Build history of the part. All positions in model axes, mm. A direction names the side the tool comes from. Give positions to 0.01 mm unless a question says otherwise; leave off trailing zeros. Order: outer loops, then holes, each group sorted by start corner. A loop starts at its lowest first (then second) coordinate and runs counter-clockwise, first axis right, second up. Notation, with made-up numbers: M -19.75,43 L 3.25,43 A22 ccw 3.25,80 Z; hole C 34.5,21.5 d10. An arc over 180 degrees is marked long. One line per item, written item: value. Start each with the question number.
from build123d import *

# Parameters (mm, degrees)
BOSS_EXTRUDE1_DEPTH = 368
SHELL2_T            = -3
BOSS_EXTRUDE3_REACH = 402.691
CUT_EXTRUDE1_REACH  = 402.691
SKETCH9_R           = 20
BOSS_EXTRUDE4_START = 10
SKETCH10_R          = 21.5
SKETCH10_R_2        = 20
BOSS_EXTRUDE4_DEPTH = 10
SKETCH11_W          = 368
SKETCH11_H          = 246
SKETCH11_W_2        = 362
SKETCH11_H_2        = 240
BOSS_EXTRUDE5_DEPTH = 38


with BuildPart() as part:
    # Sketch2 → Boss-Extrude1 (new body)
    with BuildSketch(Plane(origin=(0, 0, 0), x_dir=(0, 0, -1), z_dir=(1, 0, 0))):
        Polygon((123, -50), (-123, -50), (-52.5, 100), (52.5, 100), align=None)
    extrude(amount=BOSS_EXTRUDE1_DEPTH)

    # Shell2
    shell2_openings = [part.faces().sort_by_distance(p)[0] for p in [
        (184, 100, 0),
        (184, -50, 0),
    ]]
    offset(amount=SHELL2_T, openings=shell2_openings, kind=Kind.INTERSECTION)

    # Sketch8 → Boss-Extrude3 (add, up to next)
    with BuildSketch(Plane(origin=(368, 0, 0), x_dir=(0, 0, -1), z_dir=(1, 0, 0)), mode=Mode.PRIVATE) as boss_extrude3_sk1:
        Polygon((-4.5, 100), (-30, -35), (30, -35), (4.5, 100), (1.5, 100), (26.433333333, -32), (-26.433333333, -32), (-1.5, 100), align=None)
    boss_extrude3_tool1 = extrude(boss_extrude3_sk1.sketch, amount=-BOSS_EXTRUDE3_REACH, mode=Mode.PRIVATE) - part.part
    add(boss_extrude3_tool1.solids().sort_by_distance((368, 34.274202, 15.418325))[0])

    # Sketch9 → Cut-Extrude1 (cut, up to next)
    with BuildSketch(Plane(origin=(368, 0, 0), x_dir=(0, 0, -1), z_dir=(1, 0, 0)), mode=Mode.PRIVATE) as cut_extrude1_sk1:
        with Locations((0, -10)):
            Circle(SKETCH9_R)
    cut_extrude1_tool1 = extrude(cut_extrude1_sk1.sketch, amount=-CUT_EXTRUDE1_REACH, mode=Mode.PRIVATE) & part.part
    add(cut_extrude1_tool1.solids().sort_by_distance((368, -10, 0))[0], mode=Mode.SUBTRACT)

    # Sketch10 → Boss-Extrude4 (add)
    with BuildSketch(Plane(origin=(368, 0, 0), x_dir=(0, 0, -1), z_dir=(1, 0, 0)).offset(BOSS_EXTRUDE4_START)):
        with Locations(Location((0, -10, 0), (0, 0, 180))):
            Circle(SKETCH10_R)
        with Locations((0, -10)):
            Circle(SKETCH10_R_2, mode=Mode.SUBTRACT)
    extrude(amount=-BOSS_EXTRUDE4_DEPTH)

    # Sketch11 → Boss-Extrude5 (add)
    with BuildSketch(Plane.XZ.offset(50)):
        with Locations((184, 0)):
            Rectangle(SKETCH11_W, SKETCH11_H)
        with Locations((184, 0)):
            Rectangle(SKETCH11_W_2, SKETCH11_H_2, mode=Mode.SUBTRACT)
    extrude(amount=BOSS_EXTRUDE5_DEPTH)


solid = part.part
1) Tool access for faces 5 (the flat face through (187, -35, 0)), 6 (the flat face through (3, 20, 0)), 7 (the cylindrical face through (371.591, -27.743, -9.229)), 8 (the flat face through (378, 3, 16)), 9 (the flat face through (186.534, 31.555, -17.428)): list every direction of +Z, -Z, +X, -X, +Y, -Y with a clear straight run to the whole face (end or side of a thin tool).
2) Drop flat-ended pins along their axis: P1, Ø1, axis at y = 31.5, z = 72.5, coming from the +X side; P2, Ø1, axis at x = 196.5, y = 49, coming from the +Z side (3 decimals); P3, Ø6, axis at x = 335, y = -0.5, coming from the +Z side (3 decimals). Give the stop position or say it passes through.
3) Slice it at B-B (y = 77.5). List the corners of the cut face in (x, z) (3 decimals), plus the area to 3 significant figures.
4) Slice it at A-A (x = 167.5). List the corners of the cut face in (y, z), plus the area to 3 significant figures.
5) Slice it at D-D (y = 2). List the corners of the cut face in (x, z), plus the area to 3 significant figures.
6) Slice it at C-C (z = 84). List the corners of the cut face in (x, y), plus the area to 3 significant figures.
7) Drill centre lines: line 1 (X direction, y = -21, z = -97); line 2 (Y direction, x = 373, z = 0); line 3 (Z direction, x = 45, y = -73). Where is each one in solid material? Low to high.
8) Pull direction X, two halves, no side cores. Call faces 1 (the flat face through (365, -14, -28)), 2 (the flat face through (181, -69, 123)), 3 (the flat face through (368, -14, 26)), 4 (the flat face through (186.534, 34.924, -13.792)): pulls with the +X half, pulls with the -X half, needs draft (parallel to the pull), parting line crosses it, or undercut.
Results list:
1. face 5: -Y
1. face 6: none
1. face 7: +X
1. face 8: +Z, -Z, +X, +Y, -Y
1. face 9: +Y
2. P1: stops at x = 368
2. P2: stops at z = 76.705
2. P3: stops at z = 101.145
3. outline: M 0,-63.075 L 368,-63.075 L 368,63.075 L 0,63.075 Z; hole M 3,-59.76 L 365,-59.76 L 365,-8.75 L 3,-8.75 Z; hole M 3,-5.75 L 365,-5.75 L 365,5.75 L 3,5.75 Z; hole M 3,8.75 L 365,8.75 L 365,59.76 L 3,59.76 Z
3. area: 5,330 mm²
4. outline: M -88,-123 L -50,-123 L 100,-52.5 L 100,-49.19 L -50,-119.69 L -50,-120 L -88,-120 Z; M -88,120 L -50,120 L -50,119.69 L 100,49.19 L 100,52.5 L -50,123 L -88,123 Z; M -35,-30 L 100,-4.5 L 100,-1.5 L -32,-26.43 L -32,26.43 L 100,1.5 L 100,4.5 L -35,30 Z
4. area: 2,190 mm²
5. outline: M 0,-98.56 L 368,-98.56 L 368,-17.84 L 378,-17.84 L 378,-16 L 365,-16 L 365,-20.01 L 3,-20.01 L 3,20.01 L 365,20.01 L 365,16 L 378,16 L 378,17.84 L 368,17.84 L 368,98.56 L 0,98.56 Z; hole M 3,-95.25 L 365,-95.25 L 365,-23.01 L 3,-23.01 Z; hole M 3,23.01 L 365,23.01 L 365,95.25 L 3,95.25 Z
5. area: 5,700 mm²
6. outline: M 0,-88 L 3,-88 L 3,25.93 L 365,25.93 L 365,-88 L 368,-88 L 368,32.98 L 0,32.98 Z
6. area: 3,280 mm²
7. line 1: x = 0 to 3, 365 to 368
7. line 2: y = -31.5 to -30, 10 to 11.5
7. line 3: z = -123 to -120, 120 to 123
8. face 1: undercut
8. face 2: needs draft
8. face 3: pulls with the +X half
8. face 4: undercut
